Autodesk Inventor part; units mm, degrees
ref_plane "YZ Plane" through (0, 0, 0) normal (1, 0, 0) x (0, 1, 0)
ref_plane "XZ Plane" through (0, 0, 0) normal (0, 1, 0) x (-1, 0, 0)
ref_plane "XY Plane" through (0, 0, 0) normal (0, 0, 1) x (1, 0, 0)
sketch "Sketch1" plane through (0, 0, 0) normal (0, 0, 1) x (1, 0, 0)
  line L0 (-750, 51.8997) -> (750, 51.8997)
  line L1 (750, 51.8997) -> (750, 0)
  line L2 (750, 0) -> (-750, 0)
  line L3 (-750, 0) -> (-750, 51.8997)
  point P0 (0, 0)
  point P1 (0, 0)
  dimension "d0" = 1500
  dimension "d1" = 51.8997
extrude "Plate1" add sketch "Sketch1" along normal blind 3
sketch "Sketch2" plane through (750, 3, 0) normal (0, -1, 0) x (1, 0, 0)
  line L0 (-1500, 0) -> (0, 0)
  line L1 (0, 0) -> (0, 30)
  line L2 (0, 30) -> (-1500, 30)
  line L3 (-1500, 30) -> (-1500, 0)
edge flange "Flange1" height 30 angle 90 thickness 3 bend radius 3 thickness toward (0, -1, 0) relief tear relief width 3 relief depth 1.5 edges at (0, 0, 3) wall of the first edge with corners at (-750, 3, 0) (750, 3, 0) (750, 3, 30) (-750, 3, 30)
bend "Bend1"
corner "Corner1"
sketch "Sketch5" plane through (0, 0, 0) normal (0, 0, -1) x (-1, 0, 0)
  line L0 (750, 51.8997) -> (-750, 51.8997)
  line L1 (500, 51.8997) -> (500, 31)
  line L2 (500, 31) -> (503, 31)
  line L3 (503, 31) -> (503, 51.8997)
  line L4 (750, 0) -> (-750, 0)
  point P0 (0, 0)
  dimension "d18" = 3
  dimension "d19" = 247
  dimension "d20" = 31
extrude "Extrusion1" cut sketch "Sketch5" against normal through all
pattern_linear "Rectangular Pattern1" count 3 spacing 500 along (1, 0, 0) of "Extrusion1"
sketch "Sketch6" plane through (0, 0, 0) normal (0, 0, -1) x (-1, 0, 0)
  line L0 (-750, 51.8997) -> (-750, 6)
  circle A0 centre (-750, 51.8997) radius 15
  line L1 (-750, 51.8997) -> (-500, 51.8997)
  point P0 (0, 0)
  point P1 (-735, 51.8997)
  point P2 (-750, 36.8997)
  dimension "d24" = 30
extrude "Extrusion2" cut sketch "Sketch6" against normal through all contours L1 A0 L0 picked at (-740.1254, 50.7871)
mirror "Mirror1" about plane through (0, 0, 0) normal (1, 0, 0) of "Extrusion2"
equation "\"d1\" = Стрингер_5"
equation "\"d18\" = Thickness"
equation "\"d2\" = Thickness"
equation "\"d3\" = BendReliefWidth"
equation "\"d4\" = BendReliefDepth"
equation "\"d5\" = MinimumRemnant"
equation "\"d6\" = TransitionRadius"
equation "\"d9\" = BendRadius"
equation "\"d10\" = CornerReliefSize"
equation "\"d11\" = GapSize"
equation "\"d12\" = JacobiRadiusSize"
equation "\"BendRadius\" = Thickness"
equation "\"BendReliefWidth\" = Thickness"
equation "\"BendReliefDepth\" = 0.5 * Thickness"
equation "\"CornerReliefSize\" = 4 * Thickness"
equation "\"MinimumRemnant\" = 2 * Thickness"
equation "\"TransitionRadius\" = BendRadius"
equation "\"JacobiRadiusSize\" = BendRadius"
equation "\"GapSize\" = Thickness"
properties part number "МОО 055 стрингер борт 51"
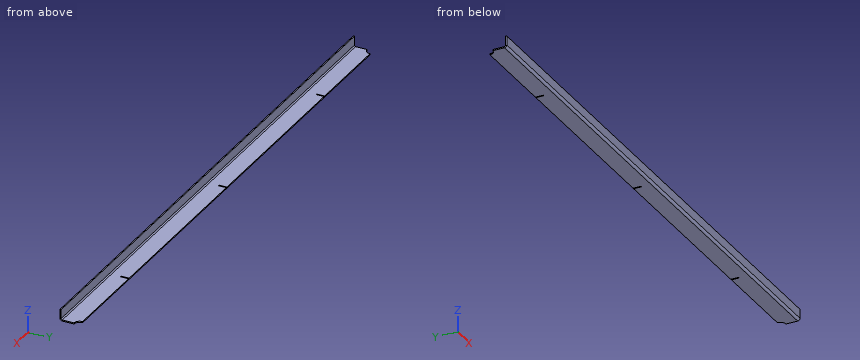
Input: part model. Units: mm. Frame: model coordinates. Coordinates: 2 decimals unless noted, no trailing zeros. Write each loop counter-clockwise with the first axis right and the second up, starting at its lowest first coordinate (ties: lowest second). Pieces come first, ordered by that corner, then holes. Notation, with made-up numbers: M -38.5,82.5 L -31.5,82.5 A18 ccw -31.5,116.5 Z; hole C -11,3 d10. An arc over 180 degrees is marked long. Answer as a JSON object with one key per item and string values. Group by question number.
(1) Ray query, line 1 along Z through (x, y) = (-237.5, 32); line 2 along Z through (x, y) = (569.5, 4.5). Return the intervals inside material, ascending. Write a range as [from, to].
(2) Section B-B on z = 21.75. Output: boundary loops of the cut face in (x, y), plus the area to 3 significant figures.
(3) Section A-A on x = 397. Output: boundary loops of the cut face in (y, z), plus the area to 3 significant figures.
(4) Contact query for flat-ended pins moving along their axis: P1, Ø1.5, axis at y = 42, z = 1, coming from the -X side; P2, Ø0.9, axis at x = 498, z = 1, coming from the +Y side; P3, Ø3.5, axis at y = 43.5, z = 1.5, coming from the +X side. Output: stop coordinate, or through.
Result set:
{
 "1": {"line 1": "z = [0, 3]", "line 2": "z = [0.19, 3.4]"},
 "2": {"outline": "M -750,0 L 750,0 L 750,3 L -750,3 Z", "area": "4,500 mm2"},
 "3": {"outline": "M 0,6 A6 ccw 6,0 L 51.9,0 L 51.9,3 L 6,3 A3 cw 3,6 L 3,30 L 0,30 Z", "area": "231 mm2"},
 "4": {"P1": "stops at x = -739.44", "P2": "stops at y = 31", "P3": "stops at x = 738.96"}
}
